Here's the drawing with two shaded views (mm, measured from the low corner). I have some questions. Give positions to 0.01 mm unless a question says otherwise; leave off trailing zeros. Loops run counter-clockwise (first coordinate to the right, second up) from the corner with the lowest first, then second, coordinate; pieces in that order, holes last.
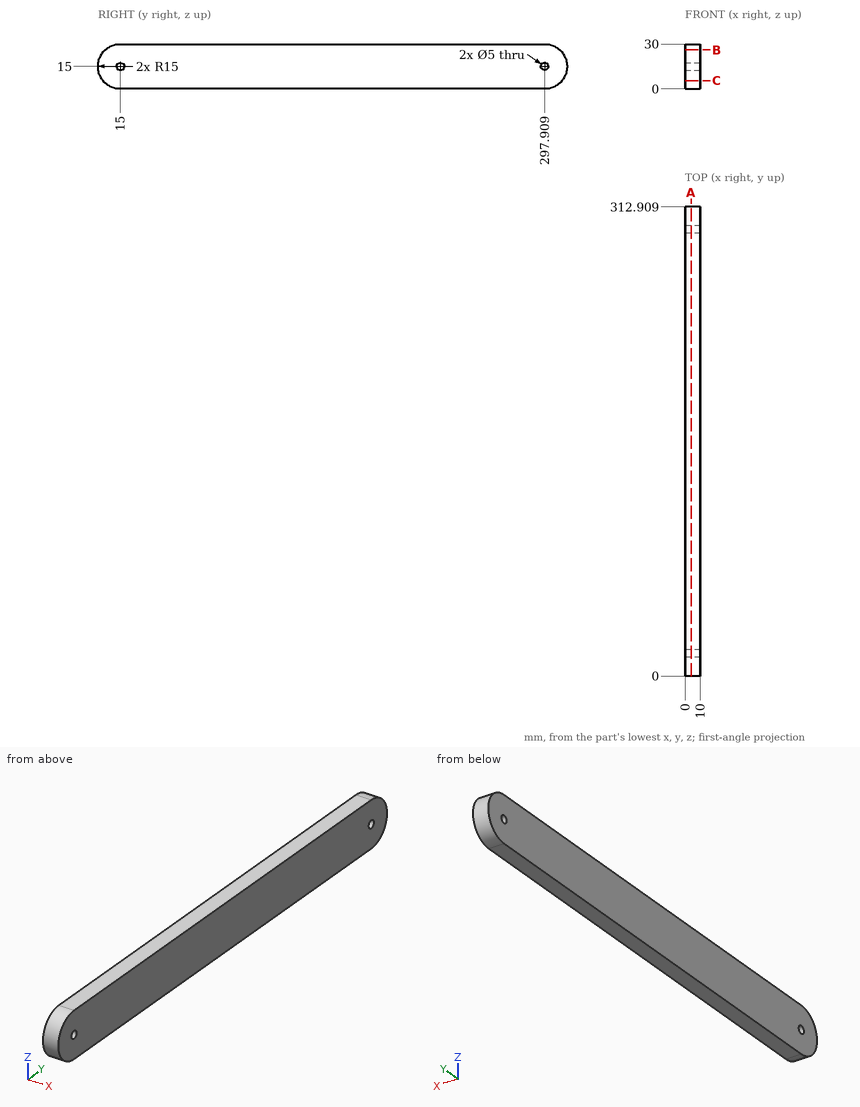
(1) Please list where these lines run through material, in increasing order: probe 1 along Y at (x, z) = (8.25, 15); probe 2 along Y at (x, z) = (2.5, 2.75); probe 3 along Y at (x, z) = (8, 10).
Returned:
probe 1: y = 0 to 12.5, 17.5 to 295.41, 300.41 to 312.91
probe 2: y = 6.34 to 306.57
probe 3: y = 0.86 to 312.05
(2) Suppose I cut it at C-C on z = 5.5. List the corners of the cut face in (x, y) for me.
Returned:
outline: (0, 3.39) - (10, 3.39) - (10, 309.52) - (0, 309.52) - close
(3) Suppose I cut it at A-A on x = 4. List the corners of the cut face in (y, z) for me.
Returned:
outline: (15, 0) - (297.91, 0) arc R15 ccw to (297.91, 30) - (15, 30) arc R15 ccw to start; hole circle Ø5 at (15, 15); hole circle Ø5 at (297.91, 15)
(4) Suppose I cut it at B-B on z = 26. List the corners of the cut face in (x, y) for me, plus the area to 3 significant figures.
Returned:
outline: (0, 4.8) - (10, 4.8) - (10, 308.11) - (0, 308.11) - close
area: 3,030 mm2
(5) Will these pins go through, and if not, where does the flat tip stop? P1, Ø5, axis at x = 7, z = 21.5, coming from the +Y side; P2, Ø5, axis at x = 8, z = 21.5, coming from the -Y side; P3, Ø4.5, axis at y = 15, z = 15, coming from the -X side; P4, Ø5, axis at x = 7.5, z = 24.5, coming from the -Y side.
Returned:
P1: stops at y = 312.37
P2: stops at y = 0.54
P3: passes through
P4: stops at y = 1.73
